```python
from build123d import *

# Parameters (mm, degrees)
SKETCH_1_W          = 40
SKETCH_1_H          = 12
SKETCH_1_R          = 1.85
EXTRUDE_1_DEPTH     = 16.1
FILLET_1_R          = 2
SKETCH_2_R          = 1.85
CUT_EXTRUDE_1_DEPTH = 20


with BuildPart() as part:
    # 草图1 → 凸台-拉伸1 (new body)
    with BuildSketch(Plane(origin=(0, 0, 0), x_dir=(1, 0, 0), z_dir=(0, 1, 0))):
        Rectangle(SKETCH_1_W, SKETCH_1_H)
        with Locations(Location((-12.5, 0, 0), (0, 0, 270))):
            Circle(SKETCH_1_R, mode=Mode.SUBTRACT)
        with Locations(Location((12.5, 0, 0), (0, 0, 270))):
            Circle(SKETCH_1_R, mode=Mode.SUBTRACT)
    extrude(amount=EXTRUDE_1_DEPTH)

    # 圆角1
    fillet_1_edges = [part.edges().sort_by_distance(p)[0] for p in [
        (20, 8.05, 6),
        (-20, 8.05, 6),
        (-20, 8.05, -6),
        (20, 8.05, -6),
    ]]
    fillet(fillet_1_edges, radius=FILLET_1_R)

    # 草图2 → 切除-拉伸1 (cut)
    with BuildSketch(Plane(origin=(0, 16.1, 0), x_dir=(1, 0, 0), z_dir=(0, 1, 0))):
        with Locations(Location((0, 0, 0), (0, 0, 270))):
            Circle(SKETCH_2_R)
    extrude(amount=-CUT_EXTRUDE_1_DEPTH, mode=Mode.SUBTRACT)


solid = part.part
```
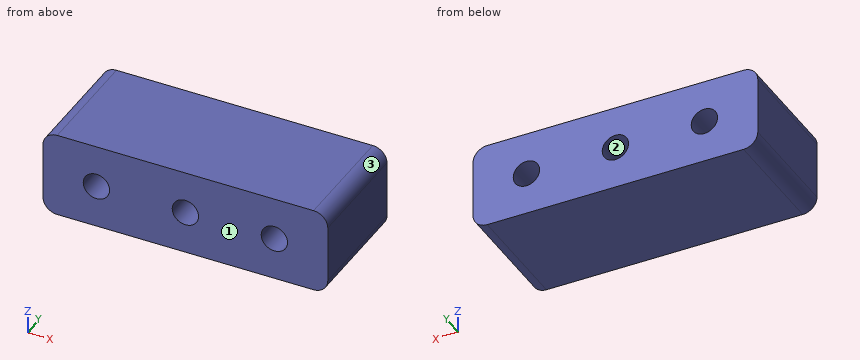
Verification items for the finished model (mm, model axes). Face numbers are marked on the shaded views. Coordinates: 2 decimals unless noted, no trailing zeros. Order: outer loops, then holes, each group sorted by start corner. A loop starts at its lowest first (then second) coordinate and runs counter-clockwise, first axis right, second up. Notation, with made-up numbers: (-27, 64.25) -> (14, 64.25) arc R10 cw to (14, 77.25) -> close; hole circle Ø1 at (0, 14.5). An arc over 180 degrees is marked (long way). Answer as CSV lines item,"result". Start each with the question number.
1) Cross-section at B-B, the plane y = 13.25. Record the boundary of the cut face in (x, z).
2) Release check for a two-part mould opening along X. For the marked faces 1, 2 and 3 record: released by +X, released by -X, zero draft, split by the parting line, or undercut.
3) Cross-section at A-A, the plane x = -12.5. Record the boundary of the cut face in (y, z), then the cut area to 3 significant figures.
4) Cross-section at C-C, the plane z = 5.25. Record the boundary of the cut face in (x, y), then the cut area to 3 significant figures.
5) Material ranges on L1, parallel to X at y = 5.25, z = 0; L2, parallel to X at y = 11.5, z = 1.5; L3, parallel to Z at x = 1, y = 8, recorded low to high. Write a range as [from, to].
Conclusion:
1,outline,"(-20, -4) arc R2 ccw to (-18, -6) -> (18, -6) arc R2 ccw to (20, -4) -> (20, 4) arc R2 ccw to (18, 6) -> (-18, 6) arc R2 ccw to (-20, 4) -> close; hole circle Ø3.7 at (-12.5, 0); hole circle Ø3.7 at (0, 0); hole circle Ø3.7 at (12.5, 0)"
2,face 1,"zero draft"
2,face 2,"undercut"
2,face 3,"released by +X"
3,outline,"(0, -6) -> (16.1, -6) -> (16.1, -1.85) -> (0, -1.85) -> close; (0, 1.85) -> (16.1, 1.85) -> (16.1, 6) -> (0, 6) -> close"
3,area,"134 mm²"
4,outline,"(-19.56, 0) -> (19.56, 0) -> (19.56, 16.1) -> (-19.56, 16.1) -> close"
4,area,"630 mm²"
5,L1,"x = [-20, -14.35], [-10.65, -1.85], [1.85, 10.65], [14.35, 20]"
5,L2,"x = [-20, -13.58], [-11.42, -1.08], [1.08, 11.42], [13.58, 20]"
5,L3,"z = [-6, -1.56], [1.56, 6]"
